Autodesk Inventor part; units mm, degrees
ref_plane "YZ Plane" through (0, 0, 0) normal (1, 0, 0) x (0, 1, 0)
ref_plane "XZ Plane" through (0, 0, 0) normal (0, 1, 0) x (-1, 0, 0)
ref_plane "XY Plane" through (0, 0, 0) normal (0, 0, 1) x (1, 0, 0)
sketch "Sketch1" plane through (0, 0, 0) normal (0, 0, 1) x (1, 0, 0)
  line L0 (0, 15.875) -> (3.175, 15.875)
  line L1 (3.175, 15.875) -> (3.175, 19.05)
  line L2 (3.175, 19.05) -> (6.35, 15.875)
  line L3 (6.35, 15.875) -> (6.35, 9.525)
  line L4 (6.35, 9.525) -> (3.175, 6.35)
  line L5 (3.175, 6.35) -> (3.175, 9.525)
  line L6 (3.175, 9.525) -> (0, 9.525)
  line L7 (9.525, 0) -> (9.525, 3.175)
  line L8 (9.525, 3.175) -> (6.35, 3.175)
  line L9 (6.35, 3.175) -> (9.525, 6.35)
  line L10 (9.525, 6.35) -> (15.875, 6.35)
  line L11 (15.875, 6.35) -> (19.05, 3.175)
  line L12 (19.05, 3.175) -> (15.875, 3.175)
  line L13 (15.875, 3.175) -> (15.875, 0)
  line L14 (25.4, 9.525) -> (22.225, 9.525)
  line L15 (22.225, 9.525) -> (22.225, 6.35)
  line L16 (22.225, 6.35) -> (19.05, 9.525)
  line L17 (19.05, 9.525) -> (19.05, 15.875)
  line L18 (19.05, 15.875) -> (22.225, 19.05)
  line L19 (22.225, 19.05) -> (22.225, 15.875)
  line L20 (22.225, 15.875) -> (25.4, 15.875)
  line L21 (15.875, 25.4) -> (15.875, 22.225)
  line L22 (15.875, 22.225) -> (19.05, 22.225)
  line L23 (19.05, 22.225) -> (15.875, 19.05)
  line L24 (15.875, 19.05) -> (9.525, 19.05)
  line L25 (9.525, 19.05) -> (6.35, 22.225)
  line L26 (6.35, 22.225) -> (9.525, 22.225)
  line L27 (9.525, 22.225) -> (9.525, 25.4)
  circle A0 centre (12.7, 12.7) radius 3.175
  line L28 (0, 23.8125) -> (0, 15.875)
  line L29 (0, 9.525) -> (0, 1.5875)
  line L30 (9.525, 0) -> (1.5875, 0)
  line L31 (15.875, 0) -> (23.8125, 0)
  line L32 (25.4, 1.5875) -> (25.4, 9.525)
  line L33 (25.4, 15.875) -> (25.4, 23.8125)
  line L34 (23.8125, 25.4) -> (15.875, 25.4)
  line L35 (9.525, 25.4) -> (1.5875, 25.4)
  arc A1 (0, 1.5875) -> (1.5875, 0) centre (1.5875, 1.5875) ccw
  arc A2 (1.5875, 25.4) -> (0, 23.8125) centre (1.5875, 23.8125) ccw
  arc A3 (25.4, 23.8125) -> (23.8125, 25.4) centre (23.8125, 23.8125) ccw
  arc A4 (23.8125, 0) -> (25.4, 1.5875) centre (23.8125, 1.5875) ccw
  point P0 (0, 0)
  point P1 (25.4, 0)
  point P2 (0, 25.4)
  dimension "d5" = 6.35
  dimension "d7" = 12.7
  dimension "d8" = 3.175
  dimension "d9" = 3.175
  dimension "d13" = 360
  dimension "d15" = 6.35
  dimension "d16" = 1.5875
extrude "Extrusion2" add sketch "Sketch1" against normal blind 127
properties part number "motor stop for turret"
The model under review builds one solid part; all positions refer to its coordinate system, in mm. A direction names the side the tool comes from. Round coordinates to 2 decimals unless told otherwise and drop trailing zeros. Loops run counter-clockwise (first coordinate to the right, second up) from the corner with the lowest first, then second, coordinate; pieces in that order, holes last. Notation, with made-up numbers: M 78.25,-10 L 94.25,-10 A13 cw 94.25,4 Z; hole C 75.5,8.5 d11. An arc over 180 degrees is marked long. Answer as CSV lines item,"result".
1. We need section A-A (x = 12.7). Give the boundary of the cut face in (y, z) (3 decimals).
Outcome:
outline,"M 6.35,-127 L 9.525,-127 L 9.525,0 L 6.35,0 Z; M 15.875,-127 L 19.05,-127 L 19.05,0 L 15.875,0 Z"
2. We need section C-C (x = 17.5). Give the boundary of the cut face in (y, z) (3 decimals).
Outcome:
outline,"M 0,-127 L 3.175,-127 L 3.175,0 L 0,0 Z; M 4.725,-127 L 20.675,-127 L 20.675,0 L 4.725,0 Z; M 22.225,-127 L 25.4,-127 L 25.4,0 L 22.225,0 Z"
3. For faces 5 (the face through (15.875, 2, -63)), 6 (the face through (19.05, 13, -63)), 7 (the face through (15.875, 24, -63)), list the 3-axis set-ups (+Z, -Z, +X, -X, +Y, -Y) from which the entire face can be reached by the end or side of a thin tool; tool diameter is ignored.
Outcome:
face 5,"+Z, -Z, -Y"
face 6,"+Z, -Z, +X"
face 7,"+Z, -Z, +Y"
4. Draft analysis for pull direction X (two halves, no side actions). For faces 1 (the face through (20, 0, -63)), 2 (the face through (17, 3.175, -63)), 3 (the face through (25.4, 20, -63)), 4 (the face through (0, 6, -63)), state which applies: pulls with the +X half, pulls with the -X half, needs draft (parallel to the pull), parting line crosses it, or undercut.
Outcome:
face 1,"needs draft"
face 2,"undercut"
face 3,"pulls with the +X half"
face 4,"pulls with the -X half"
5. To check wall thickness, follow L1, parallel to Y at x = 12.7, z = -76 (3 decimals); L2, parallel to X at y = 24, z = -8.5 (3 decimals); L3, parallel to X at y = 7.5, z = -58 (3 decimals). State the ranges of each line that lie inside material, in increasing order. Write a range as [from, to].
Outcome:
L1,"y = [6.35, 9.525], [15.875, 19.05]"
L2,"x = [0.011, 9.525], [15.875, 25.389]"
L3,"x = [0, 3.175], [4.325, 21.075], [22.225, 25.4]"
6. Insertion check: pin 1 Ø1 at (y, z) = (12.5, -92) entering from -X; pin 2 Ø1 at (y, z) = (14.5, -72) entering from +X. Each pin has a flat end and moves straight along its axis. Give the tip position at first contact, or say it passes through.
Outcome:
pin 1,"stops at x = 6.35"
pin 2,"stops at x = 19.05"
